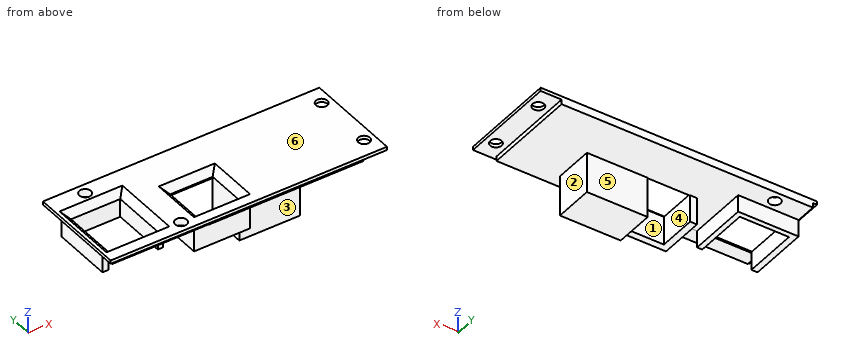
from build123d import *

# Parameters (mm, degrees)
SKIZZE1_W                       = 81.364988045
SKIZZE1_H                       = 29
AUFSATZ_LINEAR_AUSTRAGEN1_DEPTH = 1
SKIZZE2_W                       = 73.970901255
SKIZZE2_H                       = 27.9
AUFSATZ_LINEAR_AUSTRAGEN2_DEPTH = 1.385451
SKIZZE3_W                       = 17.9
SKIZZE3_H                       = 11.549624398
AUFSATZ_LINEAR_AUSTRAGEN3_DEPTH = 11.894549
SKIZZE4_W                       = 14.5
SKIZZE4_H                       = 16.1
SCHNITT_LINEAR_AUSTRAGEN1_DEPTH = 8
AUFSATZ_LINEAR_AUSTRAGEN4_DEPTH = 5
SKIZZE6_W                       = 12.5
SKIZZE6_H                       = 11.1
SCHNITT_LINEAR_AUSTRAGEN2_DEPTH = 88.193701467
AUFSATZ_LINEAR_AUSTRAGEN5_DEPTH = 8
FASE2_SIZE                      = 2
SKIZZE8_R                       = 1.7
SCHNITT_LINEAR_AUSTRAGEN3_DEPTH = 12
SCHNITT_LINEAR_AUSTRAGEN5_DEPTH = 0.114549
SKIZZE11_R                      = 1.7
SCHNITT_LINEAR_AUSTRAGEN6_DEPTH = 12
FASE3_SIZE                      = 3
SKIZZE12_R                      = 1.7
SCHNITT_LINEAR_AUSTRAGEN7_DEPTH = 88.193701467


with BuildPart() as part:
    # Skizze1 → Aufsatz-Linear austragen1 (new body)
    with BuildSketch(Plane.XY):
        with Locations((40.682494023, 14.5)):
            Rectangle(SKIZZE1_W, SKIZZE1_H)
    extrude(amount=AUFSATZ_LINEAR_AUSTRAGEN1_DEPTH)

    # Skizze2 → Aufsatz-Linear austragen2 (add)
    with BuildSketch(Plane(origin=(0, 0, 0), x_dir=(-1, 0, 0), z_dir=(0, 0, -1))):
        with Locations((-38.210114258, 15.05)):
            Rectangle(SKIZZE2_W, SKIZZE2_H)
    extrude(amount=AUFSATZ_LINEAR_AUSTRAGEN2_DEPTH)

    # Skizze3 → Aufsatz-Linear austragen3 (add)
    with BuildSketch(Plane(origin=(0, 0, -1.385450769), x_dir=(-1, 0, 0), z_dir=(0, 0, -1))):
        with Locations((-50.045564885, 10.474812199)):
            Rectangle(SKIZZE3_W, SKIZZE3_H)
    extrude(amount=AUFSATZ_LINEAR_AUSTRAGEN3_DEPTH)

    # Skizze4 → Schnitt-Linear austragen1 (cut)
    with BuildSketch(Plane(origin=(0, 0, -1.385450769), x_dir=(-1, 0, 0), z_dir=(0, 0, -1))):
        with Locations((-10.27466363, 13.35)):
            Rectangle(SKIZZE4_W, SKIZZE4_H)
    extrude(amount=-SCHNITT_LINEAR_AUSTRAGEN1_DEPTH, mode=Mode.SUBTRACT)

    # Skizze5 → Aufsatz-Linear austragen4 (add)
    with BuildSketch(Plane(origin=(0, 0, -1.385450769), x_dir=(-1, 0, 0), z_dir=(0, 0, -1))):
        Polygon((-19.02466363, 22.9), (-19.02466363, 5.3), (-17.52466363, 5.3), (-17.52466363, 21.4), (-3.02466363, 21.4), (-3.02466363, 5.3), (-1.22466363, 5.3), (-1.22466363, 22.9), align=None)
    extrude(amount=AUFSATZ_LINEAR_AUSTRAGEN4_DEPTH)

    # Skizze6 → Schnitt-Linear austragen2 (cut, through all)
    with BuildSketch(Plane(origin=(0, 0, -1.385450769), x_dir=(-1, 0, 0), z_dir=(0, 0, -1))):
        with Locations((-34.845564885, 10.55)):
            Rectangle(SKIZZE6_W, SKIZZE6_H)
    extrude(amount=-SCHNITT_LINEAR_AUSTRAGEN2_DEPTH, mode=Mode.SUBTRACT)

    # Skizze7 → Aufsatz-Linear austragen5 (add)
    with BuildSketch(Plane(origin=(0, 0, -1.385450769), x_dir=(-1, 0, 0), z_dir=(0, 0, -1))):
        Polygon((-28.595564885, 5), (-28.595564885, 16.249624398), (-26.595564885, 16.249624398), (-26.595564885, 3), (-43.095564885, 3), (-43.095564885, 16.249624398), (-41.095564885, 16.249624398), (-41.095564885, 5), align=None)
    extrude(amount=AUFSATZ_LINEAR_AUSTRAGEN5_DEPTH)

    # Fase2
    fase2_edges = [part.edges().sort_by_distance(p)[0] for p in [
        (10.27466363, 5.3, 1),
        (3.02466363, 13.35, 1),
        (10.27466363, 21.4, 1),
        (17.52466363, 13.35, 1),
        (28.595564885, 10.55, 1),
        (34.845564885, 5, 1),
        (41.095564885, 10.55, 1),
        (34.845564885, 16.1, 1),
    ]]
    chamfer(fase2_edges, length=FASE2_SIZE)

    # Skizze8 → Schnitt-Linear austragen3 (cut)
    with BuildSketch(Plane(origin=(0, 0, 0), x_dir=(-1, 0, 0), z_dir=(0, 0, -1))):
        with Locations((-78.330276465, 23.584796683)):
            Circle(SKIZZE8_R)
        with Locations((-78.330276465, 5.415203317)):
            Circle(SKIZZE8_R)
    extrude(amount=-SCHNITT_LINEAR_AUSTRAGEN3_DEPTH, mode=Mode.SUBTRACT)

    # Skizze10 → Schnitt-Linear austragen5 (cut)
    with BuildSketch(Plane(origin=(0, 0, -1.385450769), x_dir=(-1, 0, 0), z_dir=(0, 0, -1))):
        Polygon((-1.12466363, 5.3), (-26.595564885, 5.3), (-26.595564885, 1.1), (-1.22466363, 1.1), align=None)
    extrude(amount=-SCHNITT_LINEAR_AUSTRAGEN5_DEPTH, mode=Mode.SUBTRACT)

    # Skizze11 → Schnitt-Linear austragen6 (cut)
    with BuildSketch(Plane(origin=(0, 0, -1.270901539), x_dir=(-1, 0, 0), z_dir=(0, 0, -1))):
        with Locations((-22.891035352, 3.15)):
            Circle(SKIZZE11_R)
    extrude(amount=-SCHNITT_LINEAR_AUSTRAGEN6_DEPTH, mode=Mode.SUBTRACT)

    # Fase3
    # the kernel refuses this chamfer: 3 mm, written as the material it takes off along each edge
    with BuildSketch(Plane(origin=(26.595564885, 3, -1.385450769), x_dir=(0.9996219148284762, 0, -0.02749595233212696), z_dir=(0, -1, 0))) as fase3_piece_1_section:
        Polygon((FASE3_SIZE * 0.999621916941, FASE3_SIZE * 0.027495875526), (-FASE3_SIZE * 0.0274959523321, FASE3_SIZE * 0.999621914828), (0, 0), align=None)
    fase3_piece_1 = extrude(amount=9.615048972, mode=Mode.PRIVATE)
    fase3_piece_1 = split(fase3_piece_1, bisect_by=Plane(origin=(29.23101577, 2.05, -1.270901769), z_dir=(0, 0, -1)), keep=Keep.TOP, mode=Mode.PRIVATE)
    add(fase3_piece_1, mode=Mode.SUBTRACT)

    # Skizze12 → Schnitt-Linear austragen7 (cut, through all)
    with BuildSketch(Plane(origin=(0, 0, -1.385450769), x_dir=(-1, 0, 0), z_dir=(0, 0, -1))):
        with Locations((-10.32466363, 25.95)):
            Circle(SKIZZE12_R)
    extrude(amount=-SCHNITT_LINEAR_AUSTRAGEN7_DEPTH, mode=Mode.SUBTRACT)


solid = part.part
Input: part model. Units: mm. Frame: model coordinates. Face numbers are marked on the shaded views. A direction names the side the tool comes from. Give positions to 0.01 mm unless a question says otherwise; leave off trailing zeros. Loops run counter-clockwise (first coordinate to the right, second up) from the corner with the lowest first, then second, coordinate; pieces in that order, holes last. Notation, with made-up numbers: (-21, 24.5) -> (19, 24.5) arc R14 ccw to (19, 42.5) -> close; hole circle Ø3 at (58, 73). An arc over 180 degrees is marked (long way). Answer as a JSON object with one key per item and string values. Group by question number.
Item 1: Cut plane D-D, the plane x = 62. Return the cut outline in (y, z).
Item 2: Pin query (flat end, axial travel): P1, Ø2, axis at x = 28, z = -6.5, coming from the +Y side; P2, Ø1.5, axis at y = 22.5, z = -2.5, coming from the +X side; P3, Ø5, axis at y = 21.5, z = -5, coming from the -X side. Return the tip coordinate at first contact, or that it passes through.
Item 3: Cut plane C-C, the plane y = 11.25. Return the cut outline in (x, z), and give its area (3 significant figures).
Item 4: Pull-direction query (X, two-part tool) for the marked faces 1, 2, 3 and 4; classes: released by +X, released by -X, zero draft, split by the parting line, or undercut.
Item 5: Cut plane A-A, the plane z = -5. Return the cut outline in (x, y), and give its area (3 significant figures).
Item 6: Reachability of the marked faces 5 and 6 from +Z, -Z, +X, -X, +Y, -Y: full face, straight path, thin tool, end or side. Return the list, or none.
Item 7: Cut plane B-B, the plane x = 15. Return the cut outline in (y, z), and give its area (3 significant figures).
Item 8: Line query: probe 1 along X at (y, z) = (12.75, -9.25); probe 2 along X at (y, z) = (5.75, -2); probe 3 along Z at (x, y) = (71, 26.5). Output: solid intervals per line, ascending.
Checks:
{
 "1": {"outline": "(0, 0) -> (1.1, 0) -> (1.1, -1.39) -> (29, -1.39) -> (29, 1) -> (0, 1) -> close"},
 "2": {"P1": "stops at y = 16.25", "P2": "stops at x = 19.02", "P3": "stops at x = 1.22"},
 "3": {"outline": "(0, 0) -> (1.22, 0) -> (1.22, -6.39) -> (3.02, -6.39) -> (3.02, -1) -> (1.02, 1) -> (0, 1) -> close; (17.52, -6.39) -> (19.02, -6.39) -> (19.02, -1.39) -> (26.6, -1.39) -> (26.6, -9.39) -> (28.6, -9.39) -> (28.6, -1) -> (26.6, 1) -> (19.52, 1) -> (17.52, -1) -> close; (41.1, -13.28) -> (59, -13.28) -> (59, -1.39) -> (75.2, -1.39) -> (75.2, 0) -> (81.36, 0) -> (81.36, 1) -> (43.1, 1) -> (41.1, -1) -> close", "area": "357 mm²"},
 "4": {"face 1": "undercut", "face 2": "released by +X", "face 3": "zero draft", "face 4": "undercut"},
 "5": {"outline": "(1.22, 5.3) -> (3.02, 5.3) -> (3.02, 21.4) -> (17.52, 21.4) -> (17.52, 5.3) -> (19.02, 5.3) -> (19.02, 22.9) -> (1.22, 22.9) -> close; (26.6, 3) -> (43.1, 3) -> (43.1, 4.7) -> (59, 4.7) -> (59, 16.25) -> (41.1, 16.25) -> (41.1, 5) -> (28.6, 5) -> (28.6, 16.25) -> (26.6, 16.25) -> close", "area": "341 mm²"},
 "6": {"face 5": "-Z, +X, +Y", "face 6": "+Z, +X, -X, +Y, -Y"},
 "7": {"outline": "(0, 0) -> (1.1, 0) -> (1.1, -1.27) -> (5.3, -1.27) -> (5.3, -1) -> (3.3, 1) -> (0, 1) -> close; (21.4, -6.39) -> (22.9, -6.39) -> (22.9, -1.39) -> (29, -1.39) -> (29, 1) -> (23.4, 1) -> (21.4, -1) -> close", "area": "32.3 mm²"},
 "8": {"probe 1": "x = 26.6 to 28.6, 41.1 to 59", "probe 2": "x = 1.22 to 3.02, 17.52 to 19.02, 26.6 to 28.6, 41.1 to 59", "probe 3": "z = -1.39 to 1"}
}
